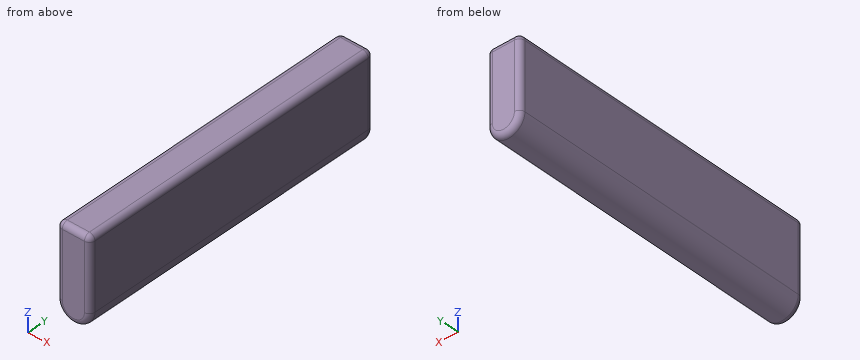
```python
from build123d import *

# Parameters (mm, degrees)
EXTRUDE_1_DEPTH = 28.4
FILLET_1_R      = 0.5


with BuildPart() as part:
    # 草图1 → 凸台-拉伸1 (new body)
    with BuildSketch(Plane(origin=(0, 0, 0), x_dir=(1, 0, 0), z_dir=(0, 1, 0))):
        with BuildLine():
            ThreePointArc((1.5, 3.25), (0, 4.75), (-1.5, 3.25))
            Line((-1.5, 3.25), (1.5, 3.25))
        make_face()
        with BuildLine():
            Line((1.5, 3.25), (-1.5, 3.25))
            ThreePointArc((-1.5, 3.25), (0, 1.75), (1.5, 3.25))
        make_face()
        with BuildLine():
            ThreePointArc((1.5, 3.25), (0, 1.75), (-1.5, 3.25))
            Line((-1.5, 3.25), (-1.5, -3.25))
            Line((-1.5, -3.25), (1.5, -3.25))
            Line((1.5, -3.25), (1.5, 3.25))
        make_face()
    extrude(amount=EXTRUDE_1_DEPTH)

    # 圆角1
    fillet_1_edges = [part.edges().sort_by_distance(p)[0] for p in [
        (-1.5, 28.4, 0),
        (0, 28.4, 3.25),
        (1.5, 28.4, 0),
        (0, 28.4, -4.75),
        (1.5, 0, 0),
        (0, 0, 3.25),
        (-1.5, 0, 0),
        (0, 0, -4.75),
        (1.5, 14.2, 3.25),
        (-1.5, 14.2, 3.25),
    ]]
    fillet(fillet_1_edges, radius=FILLET_1_R)


solid = part.part
```
Input: part model. Units: mm. Frame: model coordinates. Round coordinates to 2 decimals unless told otherwise and drop trailing zeros. Loops run counter-clockwise (first coordinate to the right, second up) from the corner with the lowest first, then second, coordinate; pieces in that order, holes last. Notation, with made-up numbers: M 39,85.25 L 49,85.25 A25 cw 49,113.25 Z; hole C 83.5,-14.75 d3. An arc over 180 degrees is marked long. Answer in a Markdown table with one row per item. Add a question column.
1. Section A-A (y = 4.5). Output: boundary loops of the cut face in (x, z).
2. Contact query for a flat-ended pin moving along its axis: pin 1 (1 mm diameter, centred on x = 0.5, y = 19, fed in from -Z). Output: stop coordinate, or through.
3. Ray query, probe 1 along Y at (x, z) = (0.4, -4.25); probe 2 along Z at (x, y) = (-0.1, 16); probe 3 along Z at (x, y) = (1.35, 11.75). Return the intervals inside material, ascending.
Values follow:
| question | item | result |
|---|---|---|
| 1 | outline | M -1.5,-3.25 A1.5 ccw 1.5,-3.25 L 1.5,2.75 A0.5 ccw 1,3.25 L -1,3.25 A0.5 ccw -1.5,2.75 Z |
| 2 | pin 1 | z = -4.75 |
| 3 | probe 1 | 0.01 to 28.39 |
| 3 | probe 2 | -4.75 to 3.25 |
| 3 | probe 3 | -3.9 to 3.11 |
